from build123d import *

# Parameters (mm, degrees)
SKETCH2_R           = 10
BOSS_EXTRUDE1_DEPTH = 15
SKETCH3_R           = 11.5
BOSS_EXTRUDE2_DEPTH = 2.3
SKETCH4_W           = 0.8
SKETCH4_H           = 4.8
BOSS_EXTRUDE3_DEPTH = 8.55
BOSS_EXTRUDE4_DEPTH = 15


with BuildPart() as part:
    # Sketch2 → Boss-Extrude1 (new body)
    with BuildSketch(Plane(origin=(0, 0, 0), x_dir=(1, 0, 0), z_dir=(0, 1, 0))):
        with Locations(Location((0, 0, 0), (0, 0, 270))):
            Circle(SKETCH2_R)
    extrude(amount=BOSS_EXTRUDE1_DEPTH)

    # Sketch3 → Boss-Extrude2 (add)
    with BuildSketch(Plane(origin=(0, 15, 0), x_dir=(1, 0, 0), z_dir=(0, 1, 0))):
        with Locations(Location((0, 0, 0), (0, 0, 270))):
            Circle(SKETCH3_R)
    extrude(amount=BOSS_EXTRUDE2_DEPTH)

    # Sketch4 → Boss-Extrude3 (add)
    with BuildSketch(Plane.XZ):
        Rectangle(SKETCH4_W, SKETCH4_H)
        with Locations((-6.8, 0)):
            Rectangle(SKETCH4_W, SKETCH4_H)
    extrude(amount=BOSS_EXTRUDE3_DEPTH)

    # Sketch5 → Boss-Extrude4 (add)
    with BuildSketch(Plane.XZ):
        with BuildLine():
            Line((-1.05, 9.944722218), (-1.05, 11.451964897))
            Line((-1.05, 11.451964897), (1.05, 11.451964897))
            Line((1.05, 11.451964897), (1.05, 9.944722218))
            ThreePointArc((1.05, 9.944722218), (0, 10), (-1.05, 9.944722218))
        make_face()
    extrude(amount=-BOSS_EXTRUDE4_DEPTH)


solid = part.part
The listing builds one solid part. Answer for the finished solid, in the listing's coordinates (mm). A direction names the side the tool comes from. Coordinates: 2 decimals unless noted, no trailing zeros. Write each loop counter-clockwise with the first axis right and the second up, starting at its lowest first coordinate (ties: lowest second). Pieces come first, ordered by that corner, then holes. Notation, with made-up numbers: M 80.5,72 L 123.5,72 A27 ccw 123.5,101 Z; hole C -34,22 d8. An arc over 180 degrees is marked long. Use one line per item in the form item = value.
Item 1: Find the intervals of material crossed by probe 1 along Y at (x, z) = (-5, -7); probe 2 along Y at (x, z) = (10, 5); probe 3 along X at (y, z) = (12.75, 10.25), in increasing order.
Model answer:
probe_1 = 0 to 17.3
probe_2 = 15 to 17.3
probe_3 = -1.05 to 1.05
Item 2: Find section D-D, the plane x = 9.5. Give the vertices of the cut face in (y, z).
Model answer:
outline = M 0,-3.12 L 15,-3.12 L 15,-6.48 L 17.3,-6.48 L 17.3,6.48 L 15,6.48 L 15,3.12 L 0,3.12 Z
Item 3: For faces 4 (the face through (0, 7, 11.452)), 5 (the face through (-7.2, -4, 0)), 6 (the face through (-1.05, 7, 11)), 7 (the face through (0, 7, -10)), 8 (the face through (-0.4, -4, 0)), determine the directions among +Z, -Z, +X, -X, +Y, -Y from which every point of the face is accessible in a straight line to the end or side of a thin tool.
Model answer:
face_4 = +Z, +X, -X, -Y
face_5 = +Z, -Z, -X, -Y
face_6 = +Z, -X, -Y
face_7 = -Y
face_8 = +Z, -Z, -Y
Item 4: Find section B-B, the plane x = 0. Give the vertices of the cut face in (y, z).
Model answer:
outline = M -8.55,-2.4 L 0,-2.4 L 0,-10 L 15,-10 L 15,-11.5 L 17.3,-11.5 L 17.3,11.5 L 15,11.5 L 15,11.45 L 0,11.45 L 0,2.4 L -8.55,2.4 Z
Item 5: Find section A-A, the plane z = 0. Give the vertices of the cut face in (x, y), plus the area to 3 significant figures.
Model answer:
outline = M -11.5,15 L -10,15 L -10,0 L -7.2,0 L -7.2,-8.55 L -6.4,-8.55 L -6.4,0 L -0.4,0 L -0.4,-8.55 L 0.4,-8.55 L 0.4,0 L 10,0 L 10,15 L 11.5,15 L 11.5,17.3 L -11.5,17.3 Z
area = 367 mm2
Item 6: The mould has two halves that part along X. Classify faces 1 (the face through (-6.4, -4, 0)), 2 (the face through (1.05, 7, 11)), 3 (the face through (5, 15, -9)): released by +X, released by -X, zero draft, split by the parting line, or undercut.
Model answer:
face_1 = undercut
face_2 = released by +X
face_3 = zero draft
Item 7: Given P1, Ø10, axis at y = 12.5, z = -6.5, coming from the +X side; P2, Ø1.4, axis at y = -6.5, z = 0.5, coming from the -X side; P3, Ø2, axis at x = 6.5, y = 0.5, coming from the +Z side; P4, Ø11.5, axis at x = 1.5, z = -4, coming from the -Y side, each flat-ended and moving along its own axis, determine where each tip first touches the part or whether it passes through.
Model answer:
P1 = 11.29
P2 = -7.2
P3 = 8.35
P4 = -8.55
Item 8: Find section C-C, the plane y = 8.5. Give the vertices of the cut face in (x, z).
Model answer:
outline = M -1.05,9.94 A10 ccw long 1.05,9.94 L 1.05,11.45 L -1.05,11.45 Z
